The listing builds one solid part. Answer for the finished solid, in the listing's coordinates (mm). Face numbers are marked on the shaded views. Give positions to 0.01 mm unless a question says otherwise; leave off trailing zeros. Write each loop counter-clockwise with the first axis right and the second up, starting at its lowest first coordinate (ties: lowest second). Pieces come first, ordered by that corner, then holes. Notation, with made-up numbers: (19.25, -33.75) -> (64.25, -33.75) arc R8 cw to (64.25, -23.75) -> close; hole circle Ø10 at (58, 43.25). An arc over 180 degrees is marked (long way). Write each question's results on one line, items separated by ' | '. Start each with the question number.
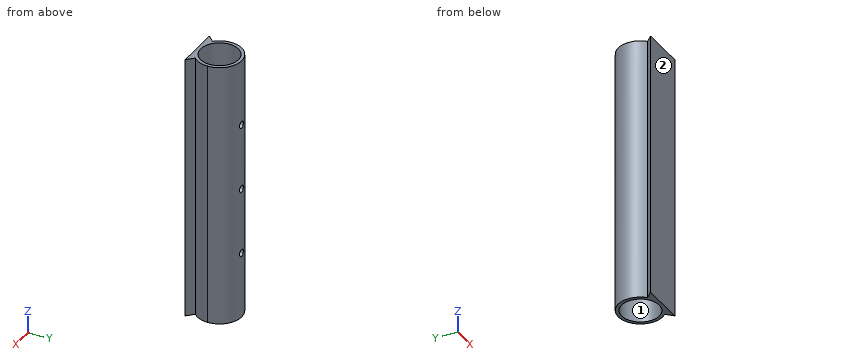
Autodesk Inventor part; units mm, degrees
ref_plane "YZ Plane" through (0, 0, 0) normal (1, 0, 0) x (0, 1, 0)
ref_plane "XZ Plane" through (0, 0, 0) normal (0, 1, 0) x (-1, 0, 0)
ref_plane "XY Plane" through (0, 0, 0) normal (0, 0, 1) x (1, 0, 0)
sketch "Sketch1" plane through (0, 0, 0) normal (0, 1, 0) x (-1, 0, 0)
  line L0 (0, 0) -> (20, 0)
  line L1 (20, 0) -> (20, -120)
  line L2 (20, -120) -> (0, -120)
  line L3 (0, -120) -> (0, 0)
  dimension "d0" = 20
  dimension "d1" = 120
extrude "Extrusion1" add sketch "Sketch1" along normal blind 20
sketch "Sketch2" plane through (0, 20, 0) normal (0, 1, 0) x (1, 0, 0)
  line L0 (-20, 120) -> (-20, 0)
  line L1 (0, 0) -> (0, 120)
  line L2 (-20, 0) -> (0, 0)
  line L3 (0, 0) -> (0, 120)
  line L4 (0, 120) -> (-20, 120)
  line L5 (-20, 120) -> (-20, 0)
  line L6 (0, 120) -> (-20, 120)
  line L7 (-20, 0) -> (-10, 0)
  line L8 (-10, 0) -> (-10, 120)
  line L9 (-10, 120) -> (-20, 120)
  line L10 (-20, 120) -> (-20, 0)
  line L11 (-10, 0) -> (-10, 60)
  line L12 (-10, 60) -> (-10, 90)
  line L13 (-10, 90) -> (-10, 30)
  circle A0 centre (-10, 30) radius 1.6
  circle A1 centre (-10, 60) radius 1.6
  circle A2 centre (-10, 90) radius 1.6
  dimension "d23" = 0
  dimension "d4" = 60
  dimension "d5" = 30
  dimension "d6" = 60
  dimension "d7" = 3.2
  dimension "d8" = 3.2
  dimension "d9" = 3.2
extrude "Extrusion2" cut sketch "Sketch2" against normal blind 35.5625 contours A2 L8 | L8 A2 | A0 L8 | L8 A0 | A1 L8 | L8 A1
sketch "Sketch3" plane through (-20, 0, 0) normal (0, 0, 1) x (1, 0, 0)
  line L0 (0, 20) -> (20, 20)
  line L1 (0, 20) -> (20, 0)
  line L2 (20, 0) -> (20, 20)
  line L3 (0, 0) -> (20, 0)
  line L4 (20, 20) -> (0, 0)
  circle A0 centre (10, 10) radius 10
  line L5 (0, 0) -> (20, 0)
  line L6 (20, 0) -> (20, -2)
  line L7 (20, -2) -> (0, -2)
  line L8 (0, -2) -> (0, 0)
  line L9 (0, 0) -> (0, 20)
  line L10 (0, 20) -> (20, 20)
  line L11 (20, 20) -> (20, 0)
  line L12 (20, 0) -> (0, 0)
  line L13 (0, 0) -> (0, 20)
  point P0 (0, 10)
  point P1 (2.9289, 2.9289)
  point P2 (10, 20)
  point P3 (20, 10)
  point P4 (17.0711, 2.9289)
  dimension "d12" = 2
extrude "Extrusion3" cut sketch "Sketch3" against normal blind 223.2 contours L0 A0 L1 | L1 A0 L9 | L0 L4 A0 | A0 L4 L9 | L2 A0 L4 | L2 L1 A0
sketch "Sketch4" plane through (-20, 0, 0) normal (0, 0, 1) x (1, 0, 0)
  arc A0 (17.0711, 2.9289) -> (2.9289, 2.9289) centre (10, 10) ccw
  circle A1 centre (10, 10) radius 10
  circle A2 centre (10, 10) radius 8.5
  point P0 (20, 0)
  dimension "d15" = 17
extrude "Extrusion4" cut sketch "Sketch4" against normal blind 267.3375 contours A2
sketch "Sketch6" plane through (0, 0, 0) normal (0, -1, 0) x (1, 0, 0)
  circle A0 centre (-10, -30) radius 1.6
  circle A1 centre (-10, -30) radius 1.6
  circle A2 centre (-10, -60) radius 1.6
  circle A3 centre (-10, -60) radius 1.6
  circle A4 centre (-10, -90) radius 1.6
  circle A5 centre (-10, -90) radius 1.6
  point P0 (0, 0)
extrude "Extrusion6" add sketch "Sketch6" against normal blind 3
sketch "Sketch7" plane through (-20, 0, 0) normal (0, 0, 1) x (1, 0, 0)
  circle A0 centre (10, 10) radius 8.5
  circle A1 centre (10, 10) radius 8.5
  point P0 (20, 0)
extrude "Extrusion7" add sketch "Sketch7" against normal blind 120
sketch "Sketch8" plane through (-20, 0, 0) normal (0, 0, 1) x (1, 0, 0)
  arc A0 (17.0711, 2.9289) -> (2.9289, 2.9289) centre (10, 10) ccw
  circle A1 centre (10, 10) radius 8.5
  point P0 (20, 0)
  dimension "d24" = 17
extrude "Extrusion8" cut sketch "Sketch8" against normal blind 241.95
properties part number "Cylinder"
1. Section D-D (y = 14) is taken. Write down the section's boundary in (x, z).
2. Section B-B (y = 5) is taken. Write down the section's boundary in (x, z), then the cut area to 3 significant figures.
3. Consider probe 1 along Z at (x, y) = (-10, 19.2); probe 2 along Y at (x, z) = (-10, -73.5); probe 3 along Y at (x, z) = (-12.5, -89.5). Determine where each line is inside the solid, lowest interval first. Write a range as [from, to].
4. Section A-A (x = -10) is taken. Write down the section's boundary in (y, z).
5. Section C-C (z = -73) is taken. Write down the section's boundary in (x, y), then the cut area to 3 significant figures.
6. Each of these flat-tipped pins is pushed along its axis until it touches: pin 1 Ø10 at (x, y) = (-10, 10) entering from -Z; pin 2 Ø1 at (x, z) = (-13, -45) entering from +Y; pin 3 Ø5 at (x, z) = (-16.5, -41.5) entering from +Y; pin 4 Ø1.5 at (y, z) = (12.5, -32) entering from -X. Where does it stop, or does it pass through?
7. The mould has two halves that part along Y. Classify the marked faces 1 and 2: pulls with the +Y half, pulls with the -Y half, needs draft (parallel to the pull), parting line crosses it, or undercut.
Results:
1) outline: (-19.17, -120) -> (-17.5, -120) -> (-17.5, 0) -> (-19.17, 0) -> close; (-2.5, -120) -> (-0.83, -120) -> (-0.83, 0) -> (-2.5, 0) -> close
2) outline: (-18.66, -120) -> (-16.87, -120) -> (-16.87, 0) -> (-18.66, 0) -> close; (-3.13, -120) -> (-1.34, -120) -> (-1.34, 0) -> (-3.13, 0) -> close | area: 429 mm²
3) probe 1: z = [-120, -91.6], [-88.4, -61.6], [-58.4, -31.6], [-28.4, 0] | probe 2: y = [0, 1.5], [18.5, 20] | probe 3: y = [0, 1.88], [18.12, 19.68]
4) outline: (0, -120) -> (1.5, -120) -> (1.5, 0) -> (0, 0) -> close; (18.5, -120) -> (20, -120) -> (20, -91.6) -> (18.5, -91.6) -> close; (18.5, -88.4) -> (20, -88.4) -> (20, -61.6) -> (18.5, -61.6) -> close; (18.5, -58.4) -> (20, -58.4) -> (20, -31.6) -> (18.5, -31.6) -> close; (18.5, -28.4) -> (20, -28.4) -> (20, 0) -> (18.5, 0) -> close
5) outline: (-20, 0) -> (0, 0) -> (-2.93, 2.93) arc R10 ccw (long way) to (-17.07, 2.93) -> close; hole circle Ø17 at (-10, 10) | area: 109 mm²
6) pin 1: passes through | pin 2: stops at y = 19.68 | pin 3: stops at y = 19.17 | pin 4: stops at x = -19.85
7) face 1: undercut | face 2: pulls with the -Y half
